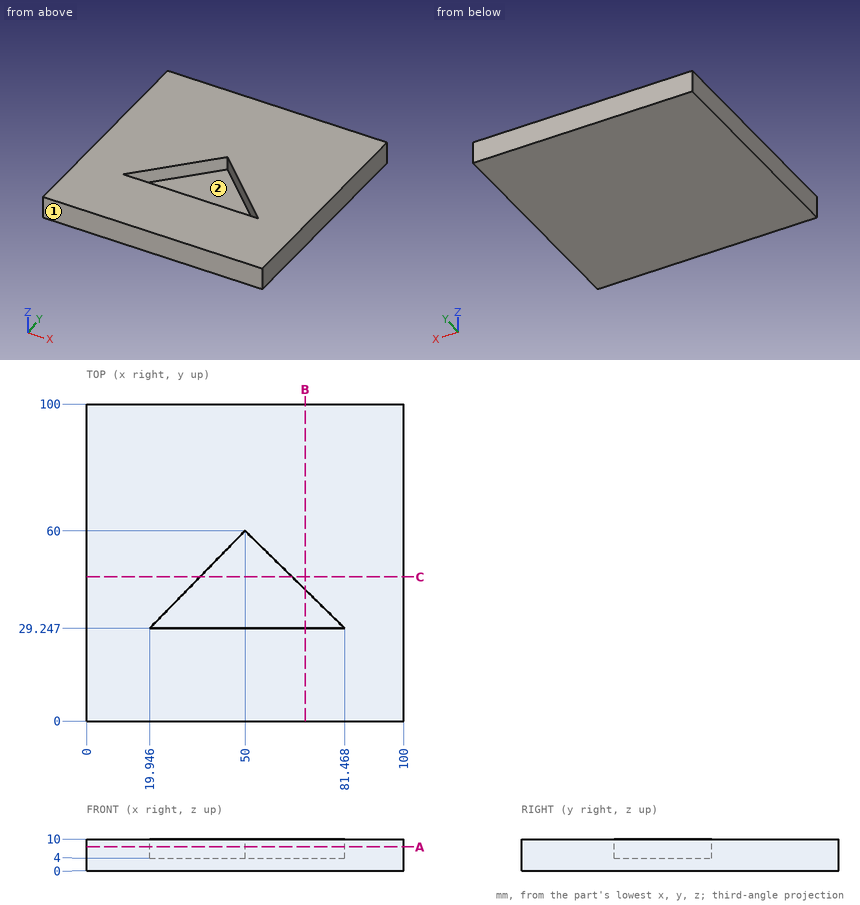
The drawing under review shows one solid part. Ordinate dimensions are in mm from its lowest x, y, z. Round coordinates to 2 decimals unless told otherwise and drop trailing zeros. Write each loop counter-clockwise with the first axis right and the second up, starting at its lowest first coordinate (ties: lowest second). Pieces come first, ordered by that corner, then holes. Notation, with made-up numbers: (42.5, -27) - (48.5, -27) arc R22 ccw to (48.5, -19) - close; hole circle Ø11 at (-4, 57). An arc over 180 degrees is marked (long way). Write each question's results on one line, items separated by ' | '.
Item 1: Take a section at C-C on y = 45.5. State the section outline as (x, z) points, then the cut area to 3 significant figures.
Calculated:
outline: (0, 0) - (100, 0) - (100, 10) - (64.84, 10) - (64.84, 4) - (35.83, 4) - (35.83, 10) - (0, 10) - close | area: 826 mm^2
Item 2: To check wall thickness, follow line 1 along X through (y, z) = (55.5, 4.5) (1 decimal); line 2 along Y through (x, z) = (35.5, 8); line 3 along X through (y, z) = (31.5, 7.5). State the ranges of each line that lie inside material, in increasing order. Write a range as from..to.
Calculated:
line 1: x = 0..45.6, 54.6..100 | line 2: y = 0..29.25, 45.16..100 | line 3: x = 0..22.15, 79.16..100
Item 3: Take a section at A-A on z = 7.5. State the section outline as (x, y) points.
Calculated:
outline: (0, 0) - (100, 0) - (100, 100) - (0, 100) - close; hole (19.95, 29.25) - (81.47, 29.25) - (50, 60) - close
Item 4: Take a section at B-B on x = 69. State the section outline as (y, z) points, then the cut area to 3 significant figures.
Calculated:
outline: (0, 0) - (100, 0) - (100, 10) - (41.43, 10) - (41.43, 4) - (29.25, 4) - (29.25, 10) - (0, 10) - close | area: 927 mm^2
Item 5: Draft analysis for pull direction X (two halves, no side actions). For the marked faces 1 and 2, state which applies: pulls with the +X half, pulls with the -X half, needs draft (parallel to the pull), parting line crosses it, or undercut.
Calculated:
face 1: needs draft | face 2: undercut
Item 6: For pin 1 (4 mm diameter, centred on x = 72.5, z = 3.5, fed in from -Y); pin 2 (9 mm diameter, centred on x = 50, y = 47, fed in from +Z), all flat-tipped, find the tip position at first contact; note any pin that passes through.
Calculated:
pin 1: stops at y = 0 | pin 2: stops at z = 4
